Input: part model. Units: mm. Frame: model coordinates. A direction names the side the tool comes from. Coordinates: 2 decimals unless noted, no trailing zeros. Order: outer loops, then holes, each group sorted by start corner. A loop starts at its lowest first (then second) coordinate and runs counter-clockwise, first axis right, second up. Notation, with made-up numbers: (63.25, 65) - (122.25, 65) arc R18 ccw to (122.25, 82) - close; hole circle Ø9 at (34.25, 46). An arc over 180 degrees is marked (long way). Use a Markdown table: item, result. Add a question column.
from build123d import *

# Parameters (mm, degrees)
EXTRUDE1_DEPTH     = 6.1722
SKETCH2_R          = 3.81
EXTRUDE2_DEPTH     = 0.8128
SKETCH3_R          = 2.2987
EXTRUDE3_DEPTH     = 2.54
SKETCH4_R          = 3.4925
EXTRUDE4_DEPTH     = 0.762
HOLE1_D            = 6.35
HOLE1_DEPTH        = 2.7686
SKETCH7_R          = 0.381
EXTRUDE5_DEPTH     = 2.2352
SKETCH8_R          = 1.7907
CUT_EXTRUDE1_DEPTH = 2.54


with BuildPart() as part:
    # Sketch1 → Extrude1 (new body)
    with BuildSketch(Plane.XY.offset(-3.3528)):
        Polygon((-4.575385413, 0), (-2.287692707, -3.9624), (2.287692707, -3.9624), (4.575385413, 0), (2.287692707, 3.9624), (-2.287692707, 3.9624), align=None)
    extrude(amount=-EXTRUDE1_DEPTH)

    # Sketch2 → Extrude2 (add)
    with BuildSketch(Plane.XY.offset(-3.3528)):
        Circle(SKETCH2_R)
    extrude(amount=EXTRUDE2_DEPTH)

    # Sketch3 → Extrude3 (add)
    with BuildSketch(Plane.XY.offset(-2.54)):
        Circle(SKETCH3_R)
    extrude(amount=EXTRUDE3_DEPTH)

    # Sketch4 → Extrude4 (add)
    with BuildSketch(Plane(origin=(0, 0, -9.525), x_dir=(-1, 0, 0), z_dir=(0, 0, -1))):
        Circle(SKETCH4_R)
    extrude(amount=EXTRUDE4_DEPTH)

    # Hole1
    with Locations(Plane(origin=(0, 0, -10.287), x_dir=(-1, 0, 0), z_dir=(0, 0, -1))):
        with Locations((0, 0)):
            Hole(HOLE1_D / 2, depth=HOLE1_DEPTH)

    # Sketch7 → Extrude5 (add)
    with BuildSketch(Plane(origin=(0, 0, -7.5184), x_dir=(-1, 0, 0), z_dir=(0, 0, -1))):
        Circle(SKETCH7_R)
    extrude(amount=EXTRUDE5_DEPTH)

    # Sketch8 → Cut-Extrude1 (cut)
    with BuildSketch(Plane.XY):
        Circle(SKETCH8_R)
    extrude(amount=-CUT_EXTRUDE1_DEPTH, mode=Mode.SUBTRACT)


solid = part.part
1) Material intervals for L1, parallel to Y at x = 0, z = -8.45 (3 decimals); L2, parallel to Y at x = 0, z = -0.55; L3, parallel to Z at x = -1.25, y = -0.5, sorted ascending.
2) Contact query for flat-ended pins moving along their axis: P1, Ø1.1, axis at x = -1, y = 0.5, coming from the +Z side; P2, Ø2.5, axis at x = -1.5, y = 1.5, coming from the +Z side; P3, Ø0.8, axis at x = 0, y = 0, coming from the -Z side; P4, Ø1, axis at x = 3.5, y = -3, coming from the -Z side. Output: stop coordinate, or through.
3) Pull-direction query (Y, two-part tool) for faces 1 (the cylindrical face through (2.123, -0.88, -1.288)), 2 (the flat face through (3.45, 1.95, -6.4)), 3 (the cylindrical face through (-0.388, -1.748, -1.252)), 4 (the flat face through (1, 0, -7.518)); classes: pulls with the +Y half, pulls with the -Y half, needs draft (parallel to the pull), parting line crosses it, or undercut.
4) Cut plane D-D (z = -7.25). Return the cut outline in (x, y).
5) Cut plane C-C (y = -1). Return the cut outline in (x, z) (3 decimals).
6) Cut plane A-A (z = -9). Return the cut outline in (x, y) (3 decimals).
7) Reachability of faces 5 (the flat face through (0, -2, 0)), 6 (the cylindrical face through (0.455, 3.463, -9.901)), 7 (the flat face through (2, -2, -2.54)) from +Z, -Z, +X, -X, +Y, -Y: full face, straight path, thin tool, end or side. Return the list, or none.
Computed:
| question | item | result |
|---|---|---|
| 1 | L1 | y = -3.962 to -3.175, -0.381 to 0.381, 3.175 to 3.962 |
| 1 | L2 | y = -2.3 to -1.79, 1.79 to 2.3 |
| 1 | L3 | z = -7.52 to -2.54 |
| 2 | P1 | stops at z = -2.54 |
| 2 | P2 | stops at z = 0 |
| 2 | P3 | stops at z = -9.75 |
| 2 | P4 | passes through |
| 3 | face 1 | parting line crosses it |
| 3 | face 2 | pulls with the +Y half |
| 3 | face 3 | undercut |
| 3 | face 4 | undercut |
| 4 | outline | (-4.58, 0) - (-2.29, -3.96) - (2.29, -3.96) - (4.58, 0) - (2.29, 3.96) - (-2.29, 3.96) - close |
| 5 | outline | (-3.998, -9.525) - (-3.346, -9.525) - (-3.346, -10.287) - (-3.013, -10.287) - (-3.013, -7.518) - (3.013, -7.518) - (3.013, -10.287) - (3.346, -10.287) - (3.346, -9.525) - (3.998, -9.525) - (3.998, -3.353) - (3.676, -3.353) - (3.676, -2.54) - (2.07, -2.54) - (2.07, 0) - (1.485, 0) - (1.485, -2.54) - (-1.485, -2.54) - (-1.485, 0) - (-2.07, 0) - (-2.07, -2.54) - (-3.676, -2.54) - (-3.676, -3.353) - (-3.998, -3.353) - close |
| 6 | outline | (-4.575, 0) - (-2.288, -3.962) - (2.288, -3.962) - (4.575, 0) - (2.288, 3.962) - (-2.288, 3.962) - close; circle Ø0.762 at (0, 0); hole circle Ø6.35 at (0, 0) |
| 7 | face 5 | +Z, +X, -X, +Y, -Y |
| 7 | face 6 | -Z |
| 7 | face 7 | +Z |
